Autodesk Fusion 360 part; units mm, degrees
sketch "Szkic1" plane through (0, 0, 0) normal (0, 0, 1) x (1, 0, 0)
  line L0 (0, 0) -> (43, 0)
  line L1 (43, 0) -> (43, 43)
  line L2 (43, 43) -> (0, 43)
  line L3 (0, 43) -> (0, 0)
  line L4 (37, 6) -> (6, 37) construction
  line L5 (6, 6) -> (37, 37) construction
  circle A0 centre (6, 37) radius 1.75
  circle A1 centre (37, 37) radius 1.75
  circle A2 centre (37, 6) radius 1.75
  circle A3 centre (6, 6) radius 1.75
  circle A4 centre (21.5, 21.5) radius 11.1
  point P0 (21.5, 21.5)
  dimension "d1" = 43
  dimension "d2" = 43
  dimension "d3" = 31
  dimension "d4" = 31
  dimension "d5" = 3.5
  dimension "d6" = 3.5
  dimension "d7" = 3.5
  dimension "d8" = 3.5
  dimension "d9" = 22.2
extrude "Wyciągnięcie proste1" add sketch "Szkic1" along normal blind 4
For this review, take the finished solid that the model builds, in its own axes (mm). Round coordinates to 2 decimals unless told otherwise and drop trailing zeros. Write each loop counter-clockwise with the first axis right and the second up, starting at its lowest first coordinate (ties: lowest second). Pieces come first, ordered by that corner, then holes. Notation, with made-up numbers: (-19, 2.25) -> (10, 2.25) arc R34 ccw to (10, 38.25) -> close; hole circle Ø9 at (-21.75, -38.5). An arc over 180 degrees is marked (long way). Use one line per item in the form item = value.
Q1. Consider section D-D (z = 2.95). State the section outline as (x, y) points.
Resolved:
outline = (0, 0) -> (43, 0) -> (43, 43) -> (0, 43) -> close; hole circle Ø3.5 at (6, 6); hole circle Ø3.5 at (6, 37); hole circle Ø22.2 at (21.5, 21.5); hole circle Ø3.5 at (37, 6); hole circle Ø3.5 at (37, 37)
Q2. Consider section B-B (y = 21.5). State the section outline as (x, z) points.
Resolved:
outline = (0, 0) -> (10.4, 0) -> (10.4, 4) -> (0, 4) -> close; (32.6, 0) -> (43, 0) -> (43, 4) -> (32.6, 4) -> close
Q3. Consider section A-A (x = 6). State the section outline as (y, z) points.
Resolved:
outline = (0, 0) -> (4.25, 0) -> (4.25, 4) -> (0, 4) -> close; (7.75, 0) -> (35.25, 0) -> (35.25, 4) -> (7.75, 4) -> close; (38.75, 0) -> (43, 0) -> (43, 4) -> (38.75, 4) -> close
Q4. To check wall thickness, follow probe 1 along Y at (x, z) = (6, 2.05); probe 2 along Y at (x, z) = (21.5, 1.3); probe 3 along Y at (x, z) = (27.5, 2.25). State the ranges of each line that lie inside material, in increasing order. Write a range as from..to.
Resolved:
probe_1 = 0..4.25, 7.75..35.25, 38.75..43
probe_2 = 0..10.4, 32.6..43
probe_3 = 0..12.16, 30.84..43
Q5. Clearance check with a flat-ended pin moving along its axis: pin 1 Ø5.5 at (x, y) = (6, 37) entering from -Z. State where the tip first meets the part, or that it passes through.
Resolved:
pin_1 = 0
Q6. The part is to be moulded in two halves that separate along X. For faces 1 (the flat face through (31, 12, 4)), 2 (the cylindrical face through (38.617, 37.67, 1.972)), 3 (the flat face through (0, 22, 2)), 4 (the cylindrical face through (31.754, 25.751, 1.972)), say which applies: released by +X, released by -X, zero draft, split by the parting line, or undercut.
Resolved:
face_1 = zero draft
face_2 = undercut
face_3 = released by -X
face_4 = undercut
